Build history of the part. All positions in model axes, mm. Face numbers are marked on the shaded views. A direction names the side the tool comes from. Round coordinates to 2 decimals unless told otherwise and drop trailing zeros. Write each loop counter-clockwise with the first axis right and the second up, starting at its lowest first coordinate (ties: lowest second). Pieces come first, ordered by that corner, then holes.
1) Saw through at A-A (y = 41). Write the cut outline in (x, z).
2) Wall check: probe 1 along Y at (x, z) = (-68.25, 1.1); probe 2 along X at (y, z) = (41, 0.7); probe 3 along Y at (x, z) = (-67.5, 2.65). Give the ranges that are in metal, low to high.
3) Saw through at D-D (y = 22). Write the cut outline in (x, z), plus the area to 3 significant figures.
4) Pull direction X, two halves, no side cores. Call the marked faces 6, 7 and 8: +X half, -X half, draft (parallel to the pull), parting line (faces both ways), or undercut.
5) Which spindle directions (+Z, -Z, +X, -X, +Y, -Y) get a long thin tool onto all of the face, cutting with end or side? Do the marked faces 1, 2, 3, 4 and 5. Say none if no direction does.
6) Saw through at C-C (y = 14.5). Write the cut outline in (x, z), plus the area to 3 significant figures.
7) Saw through at B-B (x = -71.25). Write the cut outline in (y, z), plus the area to 3 significant figures.
8) Flat gauge pins, fed straight in: pin 1 (1 mm diameter, centred on y = 31, z = 3, fed in from +X); pin 2 (1.5 mm diameter, centred on x = -70.5, z = 2, fed in from +Y); pin 3 (1.2 mm diameter, centred on y = 17, z = 2.5, fed in from +X). Where does each tip first touch, or does it go through?
from build123d import *

# Parameters (mm, degrees)
F0_R     = 2.413
F1_DEPTH = 3.96875
F2_R     = 3.81
F3_R     = 5.08


with BuildPart() as f1:
    # F0 (on Top) → F1 (new body)
    with BuildSketch(Plane.XY):
        Polygon((-63.177648, 33.202958), (-75.877648, 33.202958), (-75.877648, 43.362958), (-78.200534, 43.362958), (-78.200534, 33.202958), (-75.877648, 31.518605), (-75.877648, 7.802958), (-63.177648, 7.802958), (-63.177648, 31.518605), (-60.854763, 33.202958), (-60.854763, 43.362958), (-63.177648, 43.362958), align=None)
        with Locations((-69.527648, 16.35256)):
            Circle(F0_R, mode=Mode.SUBTRACT)
        with Locations((-69.527648, 26.51256)):
            Circle(F0_R, mode=Mode.SUBTRACT)
    extrude(amount=F1_DEPTH)

    # F2
    f2_edges = [f1.edges().sort_by_distance(p)[0] for p in [
        (-63.177648, 31.518605, 1.984375),
        (-75.877648, 31.518605, 1.984375),
        (-63.177648, 33.202958, 1.984375),
        (-75.877648, 33.202958, 1.984375),
    ]]
    fillet(f2_edges, radius=F2_R)

    # F3
    f3_edges = [f1.edges().sort_by_distance(p)[0] for p in [
        (-78.200534, 33.202958, 1.984375),
        (-60.854763, 33.202958, 1.984375),
    ]]
    fillet(f3_edges, radius=F3_R)


solid = f1.part
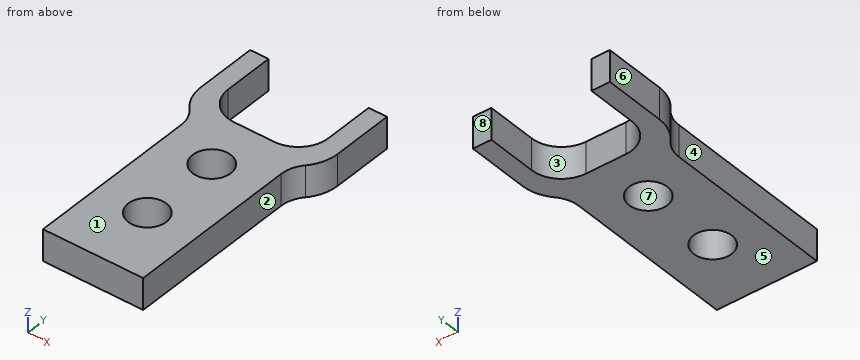
Evaluation:
1. outline: (-78.2, 0) - (-75.88, 0) - (-75.88, 3.97) - (-78.2, 3.97) - close; (-63.18, 0) - (-60.85, 0) - (-60.85, 3.97) - (-63.18, 3.97) - close
2. probe 1: y = 7.8 to 14.31, 18.4 to 24.47, 28.56 to 33.2
2. probe 2: x = -78.2 to -75.88, -63.18 to -60.85
2. probe 3: y = 7.8 to 15.04, 17.66 to 25.2, 27.82 to 33.2
3. outline: (-75.88, 0) - (-63.18, 0) - (-63.18, 3.97) - (-75.88, 3.97) - close
3. area: 50.4 mm2
4. face 6: -X half
4. face 7: undercut
4. face 8: draft
5. face 1: +Z, +X, -X, +Y, -Y
5. face 2: +Z, -Z, +X, -Y
5. face 3: +Z, -Z, +Y
5. face 4: +Z, -Z, -X, -Y
5. face 5: -Z, +X, -X, +Y, -Y
6. outline: (-75.88, 0) - (-71.07, 0) - (-71.07, 3.97) - (-75.88, 3.97) - close; (-67.98, 0) - (-63.18, 0) - (-63.18, 3.97) - (-67.98, 3.97) - close
6. area: 38.1 mm2
7. outline: (7.8, 0) - (14.66, 0) - (14.66, 3.97) - (7.8, 3.97) - close; (18.04, 0) - (24.82, 0) - (24.82, 3.97) - (18.04, 3.97) - close; (28.2, 0) - (33.2, 0) - (33.2, 3.97) - (28.2, 3.97) - close
7. area: 74.0 mm2
8. pin 1: stops at x = -62.66
8. pin 2: stops at y = 33.2
8. pin 3: stops at x = -63.18
